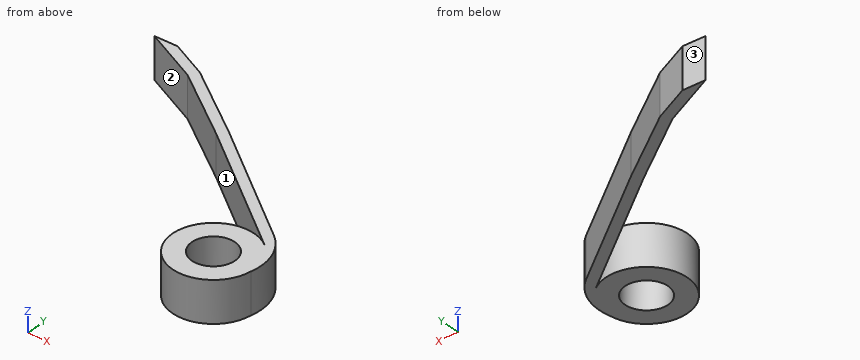
```python
from build123d import *

# Parameters (mm, degrees)
CROQUIS1_R              = 4
CROQUIS1_R_2            = 2.1
SALIENTE_EXTRUIR1_DEPTH = 4
SALIENTE_EXTRUIR3_START = -4
SALIENTE_EXTRUIR3_DEPTH = 4
REDONDEO4_R             = 5


# Read off the part's stored shape, not the designer's step: Saliente-Extruir3
with BuildPart() as part:
    # Croquis1 → Saliente-Extruir1 (new body)
    with BuildSketch(Plane.XY):
        Circle(CROQUIS1_R)
        Circle(CROQUIS1_R_2, mode=Mode.SUBTRACT)
    extrude(amount=SALIENTE_EXTRUIR1_DEPTH)

    # Saliente-Extruir3 outline → Saliente-Extruir3 (add)
    with BuildSketch(Plane.XY.offset(4).offset(SALIENTE_EXTRUIR3_START)):
        with BuildLine():
            Line((3.981796419, -0.381178801), (6.969960414, 0.948790732))
            Line((6.969960414, 0.948790732), (-9.647602311, 13.722473625))
            Line((-9.647602311, 13.722473625), (-16.604293056, 18.776920888))
            Line((-16.604293056, 18.776920888), (-20.232922351, 20.546770492))
            Line((-20.232922351, 20.546770492), (-22.514043525, 20.546770492))
            Line((-22.514043525, 20.546770492), (-17.121307849, 17.916484969))
            Line((-17.121307849, 17.916484969), (-10.246328253, 12.921405689))
            Line((-10.246328253, 12.921405689), (2.437756913, 3.171331146))
            ThreePointArc((2.437756913, 3.171331146), (3.668480336, 1.594444112), (3.981796419, -0.381178801))
        make_face()
    extrude(amount=SALIENTE_EXTRUIR3_DEPTH)

    # Redondeo4
    # the kernel refuses this fillet: 5 mm, written as the material it takes off along each edge
    with BuildSketch(Plane(origin=(6.969960414, 0.948790732, -15.212006729), x_dir=(-0.9135962080773964, -0.4066226365890155, 0), z_dir=(0, 0, 1))) as redondeo4_piece_1:
        with BuildLine():
            CenterArc((7.295339023, -2.966960117), REDONDEO4_R, 143.601912221, 64.856271299)
            Line((2.899513394, -5.349546324), (2.811596881, -5.397198048))
            Line((2.811596881, -5.397198048), (-0.087916513, -0.047651724))
            Line((-0.087916513, -0.047651724), (0, 0.1))
            ThreePointArc((0, 0.1), (1.635385507, 0.1), (3.190279653, 0.059339202))
            Line((3.190279653, 0.059339202), (3.270771013, 0))
        make_face()
    extrude(amount=34.424013457, mode=Mode.SUBTRACT)


solid = part.part
```
CAD build for the part. Positions are in the model's coordinates, mm. Face numbers are marked on the shaded views. Coordinates: 2 decimals unless noted, no trailing zeros. Order: outer loops, then holes, each group sorted by start corner. A loop starts at its lowest first (then second) coordinate and runs counter-clockwise, first axis right, second up. Notation, with made-up numbers: (86.5, 60) -> (136.5, 60) arc R20 cw to (136.5, 76) -> close; hole circle Ø1 at (79, 68). An arc over 180 degrees is marked (long way). Use one line per item in the form item = value. Start each with the question number.
1) Band-saw the part on B-B on x = 0. Give the cut face in (y, z).
2) Band-saw the part on A-A on z = 0.8. Give the cut face in (x, y), then the cut area to 3 significant figures.
3) Drop flat-ended pins along their axis: pin 1 (1.5 mm diameter, centred on y = 2.5, z = 2, fed in from -X); pin 2 (2 mm diameter, centred on y = 7.5, z = 3, fed in from -X); pin 3 (1 mm diameter, centred on y = 17.5, z = 1, fed in from -X). Give the stop position or say it passes through.
4) Band-saw the part on C-C on y = 0. Give the cut face in (x, z), then the cut area to 3 significant figures.
5) Band-saw the part on D-D on x = -7.25. Give the cut face in (y, z), then the cut area to 3 significant figures.
6) Pull direction Y, two halves, no side cores. Call the marked faces 1, 2 and 3: +Y half, -Y half, draft (parallel to the pull), parting line (faces both ways), or undercut.
7) Drill centre lines: L1, parallel to Y at x = 0, z = 2.05; L2, parallel to Y at x = -2.25, z = 0.95; L3, parallel to X at y = 6.5, z = 3.25. Where is each one in solid material? Low to high. Write a range as [from, to].
Entries:
q1.outline = (-4, 0) -> (-2.1, 0) -> (-2.1, 4) -> (-4, 4) -> close; (2.1, 0) -> (4, 0) -> (4, 4) -> (2.1, 4) -> close; (5.05, 0) -> (6.31, 0) -> (6.31, 4) -> (5.05, 4) -> close
q2.outline = (-22.51, 20.55) -> (-17.12, 17.92) -> (-10.25, 12.92) -> (2.44, 3.17) arc R4 ccw (long way) to (3.98, -0.38) arc R5 ccw to (2.15, 4.66) -> (-9.65, 13.72) -> (-16.6, 18.78) -> (-20.23, 20.55) -> close; hole circle Ø4.2 at (0, 0)
q2.area = 67.6 mm2
q3.pin_1 = -3.6
q3.pin_2 = -4.49
q3.pin_3 = -17.29
q4.outline = (-4, 0) -> (-2.1, 0) -> (-2.1, 4) -> (-4, 4) -> close; (2.1, 0) -> (4.05, 0) -> (4.05, 4) -> (2.1, 4) -> close
q4.area = 15.4 mm2
q5.outline = (10.62, 0) -> (11.88, 0) -> (11.88, 4) -> (10.62, 4) -> close
q5.area = 5.05 mm2
q6.face_1 = undercut
q6.face_2 = -Y half
q6.face_3 = +Y half
q7.L1 = [-4, -2.1], [2.1, 4], [5.05, 6.31]
q7.L2 = [-3.31, 3.31], [6.77, 8.04]
q7.L3 = [-1.89, -0.25]
